Autodesk Inventor part; units mm, degrees
ref_plane "YZ Plane" through (0, 0, 0) normal (1, 0, 0) x (0, 1, 0)
ref_plane "XZ Plane" through (0, 0, 0) normal (0, 1, 0) x (-1, 0, 0)
ref_plane "XY Plane" through (0, 0, 0) normal (0, 0, 1) x (1, 0, 0)
sketch "Sketch1" plane through (0, 0, 0) normal (0, 0, 1) x (1, 0, 0)
  circle A0 centre (0, 0) radius 4
  line L0 (15, 1) -> (15, 4)
  line L1 (4, 0) -> (7.8423, 0)
  line L2 (15, 4) -> (0, 4)
  line L3 (15, -1) -> (15, -4)
  line L4 (15, -4) -> (0, -4)
  line L5 (15, 1) -> (15, -1)
  point P0 (0, -4)
  dimension "d0" = 8
  dimension "d2" = 15
extrude "Extrusion1" add sketch "Sketch1" along normal mid plane 10 contours A0 L2 L0 L5 L3 L4
extrude "Extrusion2" add sketch "Sketch1" along normal mid plane 20 contours A0
sketch "Sketch2" plane through (15, -4, 5) normal (1, 0, 0) x (0, 0, -1)
  circle A0 centre (5, 4) radius 2.5
  line L0 (0, 0) -> (0, 8)
  line L1 (10, 8) -> (10, 0)
  line L2 (0, 8) -> (10, 8)
  line L3 (10, 8) -> (10, 0)
  line L4 (10, 0) -> (0, 0)
  line L5 (0, 0) -> (0, 8)
  dimension "d7" = 5
extrude "Extrusion3" add sketch "Sketch2" along normal blind 5
properties part number "Pitch and Yaw"
Input: part model. Units: mm. Frame: model coordinates. A direction names the side the tool comes from. Give positions to 0.01 mm unless a question says otherwise; leave off trailing zeros. Write each loop counter-clockwise with the first axis right and the second up, starting at its lowest first coordinate (ties: lowest second). Pieces come first, ordered by that corner, then holes. Notation, with made-up numbers: M 82.5,27.5 L 115.5,27.5 A31 ccw 115.5,65.5 Z; hole C 27,57.25 d4. An arc over 180 degrees is marked long. Use one line per item in the form item = value.
1. Ray query, L1, parallel to Y at x = 16.1, z = 0; L2, parallel to Z at x = 12.75, y = 3.25; L3, parallel to X at y = 0, z = -7. Return the intervals inside material, ascending.
Outcome:
L1 = -4 to -2.5, 2.5 to 4
L2 = -5 to 5
L3 = -4 to 4
2. First-contact query: P1, Ø2.5, axis at x = 14, y = -1.5, coming from the +Z side; P2, Ø1, axis at x = 9, y = -1.5, coming from the -Z side; P3, Ø1.5, axis at y = 0.5, z = 1, coming from the +X side. Flat tips, straight axial feed; report the tip coordinate or a pass-through.
Outcome:
P1 = 5
P2 = -5
P3 = 15
3. Cut plane C-C on z = -1.75. Return loops of the section in (x, y).
Outcome:
outline = M 0,-4 L 20,-4 L 20,-1.79 L 15,-1.79 L 15,1.79 L 20,1.79 L 20,4 L 0,4 A4 ccw Z
4. Cut plane D-D on y = 1.5. Return loops of the section in (x, z), and give its area (3 significant figures).
Outcome:
outline = M -3.71,-10 L 3.71,-10 L 3.71,-5 L 20,-5 L 20,-2 L 15,-2 L 15,2 L 20,2 L 20,5 L 3.71,5 L 3.71,10 L -3.71,10 Z
area = 291 mm²
5. Reachability of faces 1 (the face through (-4, 0, 0)), 2 (the face through (17.46, 2.44, 0.54)), 3 (the face through (0, 0, 10)) from +Z, -Z, +X, -X, +Y, -Y: full face, straight path, thin tool, end or side. Return the list, or none.
Outcome:
face_1 = none
face_2 = +X
face_3 = +Z, +X, -X, +Y, -Y
6. Cut plane A-A on x = 18.75. Return loops of the section in (y, z).
Outcome:
outline = M -4,-5 L 4,-5 L 4,5 L -4,5 Z; hole C 0,0 d5
7. Mould query, pull axis Z, two halves, no side actions, for faces 4 (the face through (10, 4, 0)), 5 (the face through (15, 0, 0)), 6 (the face through (0, 0, -10)). Classes: released by +Z, released by -Z, zero draft, split by the parting line, or undercut.
Outcome:
face_4 = zero draft
face_5 = undercut
face_6 = released by -Z
8. Cut plane B-B on y = 0. Return loops of the section in (x, z).
Outcome:
outline = M -4,-10 L 4,-10 L 4,-5 L 20,-5 L 20,-2.5 L 15,-2.5 L 15,2.5 L 20,2.5 L 20,5 L 4,5 L 4,10 L -4,10 Z
